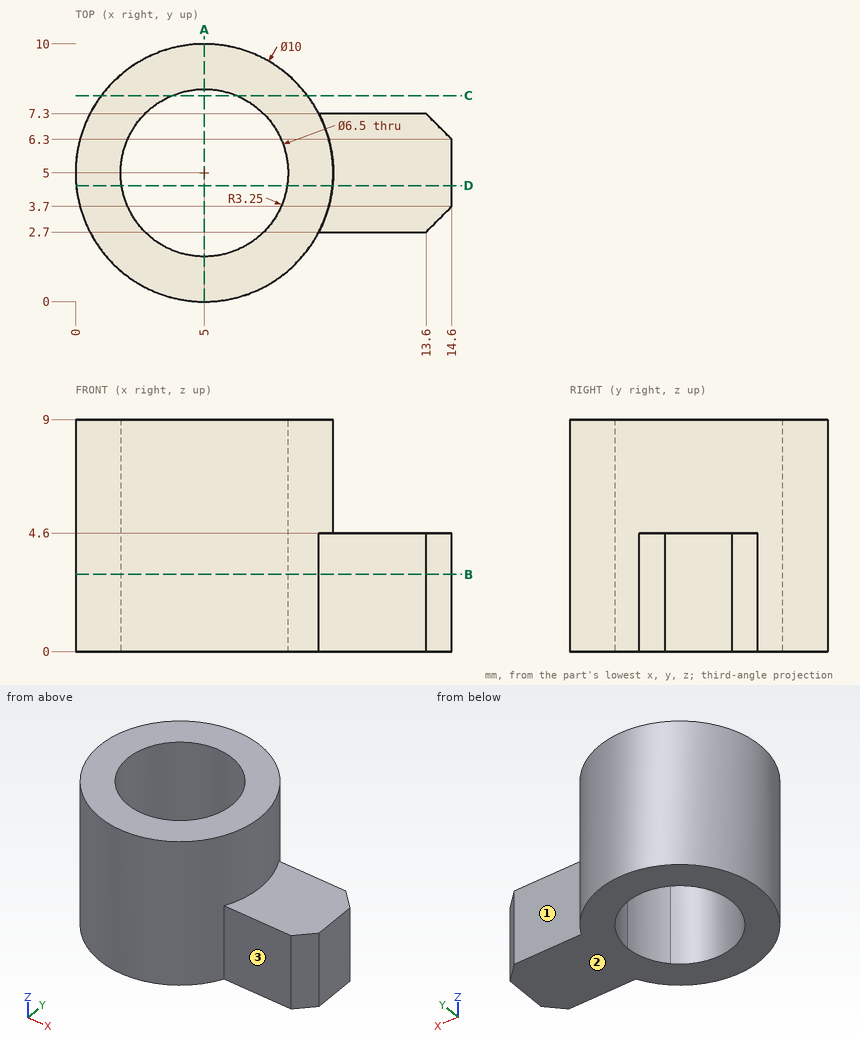
Answer from the drawing. Dimensions are ordinates in mm from the lowest x, y and z of the part. A direction names the side the tool comes from. Give positions to 0.01 mm unless a question says otherwise; leave off trailing zeros. Loops run counter-clockwise (first coordinate to the right, second up) from the corner with the lowest first, then second, coordinate; pieces in that order, holes last. Notation, with made-up numbers: (56.25, 25) - (100.25, 25) arc R10 cw to (100.25, 44) - close; hole circle Ø11 at (82, 65). An arc over 180 degrees is marked (long way). Answer as CSV lines item,"result". Start each with the question number.
Item 1: A cutting plane is placed at B-B on z = 3. Determine the outline of the cut face in (x, y), then the cut area to 3 significant figures.
Item 2: A cutting plane is placed at C-C on y = 8. Determine the outline of the cut face in (x, z).
Item 3: Each of these flat-tipped pins is pushed along its axis until it touches: pin 1 (3 mm diameter, centred on x = 9.5, z = 5.5, fed in from -Y); pin 2 (1 mm diameter, centred on x = 6, z = 5, fed in from -Y); pin 3 (1.4 mm diameter, centred on x = 12.5, y = 4, fed in from +Z). Where does it stop, or does it pass through?
Item 4: A cutting plane is placed at D-D on y = 4.5. Determine the outline of the cut face in (x, z).
Item 5: Find the intervals of material crossed by line 1 (X direction, y = 5, z = 6.75); line 2 (X direction, y = 5, z = 2), in increasing order. Write a range as from..to.
Item 6: For the marked faces 1, 2 and 3, determine the directions among +Z, -Z, +X, -X, +Y, -Y from which every point of the face is accessible in a straight line to the end or side of a thin tool.
Item 7: A cutting plane is placed at A-A on x = 5. Determine the outline of the cut face in (y, z).
Found:
1,outline,"(9.44, 2.7) - (13.6, 2.7) - (14.6, 3.7) - (14.6, 6.3) - (13.6, 7.3) - (9.44, 7.3) arc R5 ccw (long way) to start; hole circle Ø6.5 at (5, 5)"
1,area,"66.4 mm^2"
2,outline,"(1, 0) - (3.75, 0) - (3.75, 9) - (1, 9) - close; (6.25, 0) - (9, 0) - (9, 9) - (6.25, 9) - close"
3,pin 1,"stops at y = 1"
3,pin 2,"stops at y = 0.03"
3,pin 3,"stops at z = 4.6"
4,outline,"(0.03, 0) - (1.79, 0) - (1.79, 9) - (0.03, 9) - close; (8.21, 0) - (14.6, 0) - (14.6, 4.6) - (9.97, 4.6) - (9.97, 9) - (8.21, 9) - close"
5,line 1,"x = 0..1.75, 8.25..10"
5,line 2,"x = 0..1.75, 8.25..14.6"
6,face 1,"+Z, -Z, +X, +Y"
6,face 2,"-Z, +X, -X, +Y, -Y"
6,face 3,"+Z, -Z, +X, -Y"
7,outline,"(0, 0) - (1.75, 0) - (1.75, 9) - (0, 9) - close; (8.25, 0) - (10, 0) - (10, 9) - (8.25, 9) - close"
